For this review, take the finished solid that the model builds, in its own axes (mm). Coordinates: 2 decimals unless noted, no trailing zeros. Order: outer loops, then holes, each group sorted by start corner. A loop starts at its lowest first (then second) coordinate and runs counter-clockwise, first axis right, second up. Notation, with made-up numbers: (61, -14.5) -> (119, -14.5) arc R16 ccw to (119, 7.5) -> close; hole circle Ø8 at (75.25, 63). An arc over 180 degrees is marked (long way). Answer as a JSON object with one key per item and string values. Group by question number.
1) Add section A-A, the plane x = 160. Write out the cut boundary in (y, z), then the cut area to 3 significant figures.
2) Add section B-B, the plane z = 104. Write out the cut boundary in (x, y) (3 decimals), then the cut area to 3 significant figures.
3) Wall thickness on L1, parallel to X at y = 4, z = 98.5 (3 decimals); L2, parallel to Z at x = 137, y = 2.25 (3 decimals); L3, parallel to Z at x = 144, y = 2: over which ranges is each line inside the solid? List them lowest first.
4) For pin 1 (3 mm diameter, centred on x = 48.5, y = 2, fed in from +Z); pin 2 (2 mm diameter, centred on y = 0.5, z = 84.5, fed in from -X) (3 decimals); pin 3 (7.5 mm diameter, centred on x = 127, z = -17.145, fed in from +Y); pin 4 (3 mm diameter, centred on y = 3.5, z = 60, fed in from +X) (3 decimals), all flat-tipped, find the tip position at first contact; note any pin that passes through.
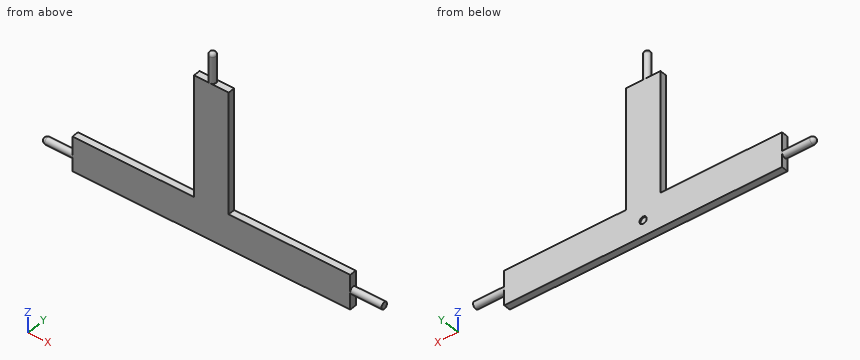
Autodesk Inventor part; units mm, degrees
ref_plane "YZ Plane" through (0, 0, 0) normal (1, 0, 0) x (0, 1, 0)
ref_plane "XZ Plane" through (0, 0, 0) normal (0, 1, 0) x (-1, 0, 0)
ref_plane "XY Plane" through (0, 0, 0) normal (0, 0, 1) x (1, 0, 0)
sketch "Sketch1" plane through (0, 0, 0) normal (0, 1, 0) x (-1, 0, 0)
  line L0 (-254, 0) -> (-254, -31.75)
  line L1 (-254, -31.75) -> (0, -31.75)
  line L2 (0, -31.75) -> (0, 0)
  line L3 (-111.125, -15.875) -> (-142.875, -15.875)
  line L4 (-142.875, 0) -> (-142.875, 111.125)
  line L5 (-142.875, 111.125) -> (-111.125, 111.125)
  line L6 (-111.125, 111.125) -> (-111.125, 0)
  line L7 (0, 0) -> (-111.125, 0)
  line L8 (-142.875, 0) -> (-254, 0)
  point P0 (-127, -15.875)
  dimension "d0" = 254
  dimension "d1" = 31.75
  dimension "d5" = 15.875
  dimension "d6" = 127
  dimension "d7" = 15.875
  dimension "d8" = 127
extrude "Extrusion1" add sketch "Sketch1" along normal blind 6.35
sketch "Sketch3" plane through (0, 6.35, 0) normal (0, 1, 0) x (1, 0, 0)
  line L0 (0, 0) -> (111.125, 0)
  line L1 (0, 31.75) -> (0, 0)
  circle A0 centre (127, 17.145) radius 3.3156
  dimension "d13" = 17.145
  dimension "d14" = 127
extrude "Extrusion3" cut sketch "Sketch3" against normal blind 1.27
sketch "Sketch4" plane through (254, 0, 0) normal (1, 0, 0) x (0, 0, -1)
  line L0 (31.75, 0) -> (0, 0)
  line L1 (31.75, 0) -> (31.75, 6.35)
  circle A0 centre (15.875, 3.175) radius 3.175
  dimension "d21" = 15.875
  dimension "d22" = 3.175
extrude "Extrusion4" add sketch "Sketch4" along normal blind 28.575
pattern_circular "Circular Pattern2" count 3 over 180 about axis through (127, 6.35, -17.145) along (0, -1, 0) of "Extrusion4"
fillet "Fillet1" radius 3.175 1 edges at (122.555, 3.175, 138.43)
fillet "Fillet2" radius 3.175 1 edges at (-28.575, 3.175, -21.59)
properties part number "Motor_Mount"
Output values:
{
 "1": {"outline": "(0, -31.75) -> (6.35, -31.75) -> (6.35, 0) -> (0, 0) -> close", "area": "202 mm²"},
 "2": {"outline": "(111.125, 0) -> (142.875, 0) -> (142.875, 6.35) -> (111.125, 6.35) -> close", "area": "202 mm²"},
 "3": {"L1": "x = 111.125 to 142.875", "L2": "z = -31.75 to 111.125", "L3": "z = -31.75 to 0"},
 "4": {"pin 1": "stops at z = 0", "pin 2": "stops at x = 111.125", "pin 3": "stops at y = 6.35", "pin 4": "stops at x = 142.875"}
}
